from build123d import *

# Parameters (mm, degrees)
SKETCH2_R               = 3.5
SKETCH2_R_2             = 2.5
BOSS_EXTRUDE1_DEPTH     = 10
CUT_EXTRUDE1_DEPTH      = 85.683624036
CUT_EXTRUDE1_DEPTH_BACK = 85.683624036
SKETCH3_R               = 2.5
FILLET1_R               = 2


with BuildPart() as part:
    # Sketch1 → Revolve1 (revolve)
    with BuildSketch(Plane(origin=(0, 0, 0), x_dir=(0, 0, -1), z_dir=(1, 0, 0)), mode=Mode.PRIVATE) as revolve1_sk:
        with BuildLine():
            Line((0, 0), (0, 52.809927725))
            ThreePointArc((0, 52.809927725), (0.130798304, 53.244522907), (0.479738309, 53.534733247))
            Line((0.479738309, 53.534733247), (0.872854821, 53.701601306))
            ThreePointArc((0.872854821, 53.701601306), (1.6002, 54.8005), (0.872854821, 55.899398694))
            Line((0.872854821, 55.899398694), (0.479738309, 56.066266753))
            ThreePointArc((0.479738309, 56.066266753), (0.130798304, 56.356477093), (0, 56.791072275))
            Line((0, 56.791072275), (0, 59.4614))
            Line((0, 59.4614), (2.8448, 59.4614))
            Line((2.8448, 59.4614), (7.9248, 45.504214709))
            Line((7.9248, 45.504214709), (7.9248, 0))
            Line((7.9248, 0), (0, 0))
        make_face()
    revolve(revolve1_sk.sketch.rotate(Axis((0, 0, 0), (0, 0, -1)), 90), axis=Axis((0, 0, 0), (0, 0, -1)))

    # Sketch2 → Boss-Extrude1 (add)
    with BuildSketch(Plane(origin=(0, 0, -7.9248), x_dir=(-1, 0, 0), z_dir=(0, 0, -1))):
        with Locations(Location((0, 0, 0), (0, 0, 180))):
            Circle(SKETCH2_R)
        Circle(SKETCH2_R_2, mode=Mode.SUBTRACT)
    extrude(amount=BOSS_EXTRUDE1_DEPTH)

    # Sketch3 → Cut-Extrude1 (cut, two sides: drawn at the far end of the back side and taken through both)
    with BuildSketch(Plane(origin=(0, 0, -7.9248), x_dir=(-1, 0, 0), z_dir=(0, 0, -1)).offset(-CUT_EXTRUDE1_DEPTH_BACK)):
        Circle(SKETCH3_R)
    extrude(amount=CUT_EXTRUDE1_DEPTH + CUT_EXTRUDE1_DEPTH_BACK, mode=Mode.SUBTRACT)

    # Fillet1
    fillet1_edges = [part.edges().sort_by_distance(p)[0] for p in [
        (-3.5, 0, -7.9248),
    ]]
    fillet(fillet1_edges, radius=FILLET1_R)


solid = part.part
Build history of the part. All positions in model axes, mm. Coordinates: 2 decimals unless noted, no trailing zeros. Order: outer loops, then holes, each group sorted by start corner. A loop starts at its lowest first (then second) coordinate and runs counter-clockwise, first axis right, second up. Notation, with made-up numbers: (6.5, -30) - (29.5, -30) arc R18 cw to (29.5, -17) - close; hole circle Ø10 at (42, 72). An arc over 180 degrees is marked (long way). Put each result on its own line as item: value.
1. Pull direction X, two halves, no side cores. Call faces 1 (the face through (3.233, 1.341, -13.869)), 2 (the face through (2, 2, -17.925)), 3 (the face through (0.54, -2.44, -8.84)): pulls with the +X half, pulls with the -X half, needs draft (parallel to the pull), parting line crosses it, or undercut.
Answer sheet:
face 1: parting line crosses it
face 2: needs draft
face 3: undercut
2. Saw through at A-A (x = 0). Write the cut outline in (y, z), and give its area (3 significant figures).
Answer sheet:
outline: (-59.46, -2.84) - (-45.5, -7.92) - (-5.5, -7.92) arc R2 cw to (-3.5, -9.92) - (-3.5, -17.92) - (-2.5, -17.92) - (-2.5, 0) - (-52.81, 0) arc R0.79 ccw to (-53.53, -0.48) - (-53.7, -0.87) arc R1.19 cw to (-55.9, -0.87) - (-56.07, -0.48) arc R0.79 ccw to (-56.79, 0) - (-59.46, 0) - close; (2.5, -17.92) - (3.5, -17.92) - (3.5, -9.92) arc R2 cw to (5.5, -7.92) - (45.5, -7.92) - (59.46, -2.84) - (59.46, 0) - (56.79, 0) arc R0.79 ccw to (56.07, -0.48) - (55.9, -0.87) arc R1.19 cw to (53.7, -0.87) - (53.53, -0.48) arc R0.79 ccw to (52.81, 0) - (2.5, 0) - close
area: 847 mm^2
3. Drop flat-ended pins along their axis: P1, Ø3, axis at x = 0, y = 0, coming from the -Z side; P2, Ø4, axis at x = -10, z = -3, coming from the -Y side. Give the stop position or say it passes through.
Answer sheet:
P1: passes through
P2: stops at y = -58.92
4. Saw through at C-C (z = -15.25). Write the cut outline in (x, y), and give its area (3 significant figures).
Answer sheet:
outline: circle Ø7 at (0, 0); hole circle Ø5 at (0, 0)
area: 18.8 mm^2
5. Probe line 1 along Z through (x, y) = (3.5, 10); line 2 along Y through (x, z) = (0, -9); line 3 along Y through (x, z) = (0, -10.75). List the from-to ranges inside material, lowest first. Write a range as [from, to].
Answer sheet:
line 1: z = [-7.92, 0]
line 2: y = [-3.73, -2.5], [2.5, 3.73]
line 3: y = [-3.5, -2.5], [2.5, 3.5]
